```python
from build123d import *

# Parameters (mm, degrees)
SKETCH2_W           = 65
SKETCH2_H           = 65
BOSS_EXTRUDE1_DEPTH = 7
SKETCH3_R           = 5
BOSS_EXTRUDE2_DEPTH = 15
SKETCH4_R           = 4
CUT_EXTRUDE1_DEPTH  = 49.347699015


with BuildPart() as part:
    # Sketch2 → Boss-Extrude1 (new body)
    with BuildSketch(Plane.XY):
        Rectangle(SKETCH2_W, SKETCH2_H)
    extrude(amount=BOSS_EXTRUDE1_DEPTH)

    # Sketch3 → Boss-Extrude2 (add)
    with BuildSketch(Plane.XY.offset(7)):
        with Locations(Location((0, 0, 0), (0, 0, 180))):
            Circle(SKETCH3_R)
    extrude(amount=BOSS_EXTRUDE2_DEPTH)

    # Sketch4 → Cut-Extrude1 (cut, through all)
    with BuildSketch(Plane.XY.offset(7)):
        with Locations((-27.162431983, 27.037591963)):
            Circle(SKETCH4_R)
    extrude(amount=-CUT_EXTRUDE1_DEPTH, mode=Mode.SUBTRACT)


solid = part.part
```
Source: CAD feature listing. Evaluate the final solid. Frame: model axes, mm. A direction names the side the tool comes from. Round coordinates to 2 decimals unless told otherwise and drop trailing zeros. Order: outer loops, then holes, each group sorted by start corner. A loop starts at its lowest first (then second) coordinate and runs counter-clockwise, first axis right, second up. Notation, with made-up numbers: (72, 40) -> (107, 40) arc R16 cw to (107, 50) -> close; hole circle Ø7 at (69, 48). An arc over 180 degrees is marked (long way). One line per item, written item: value. Start each with the question number.
Q1. Section query C-C (x = -27). Return the cut outline in (y, z).
Q2. Material intervals for probe 1 along Z at (x, y) = (-19, -26); probe 2 along X at (y, z) = (24, 4.5); probe 3 along X at (y, z) = (4, 17.5), sorted ascending.
Q3. Pin query (flat end, axial travel): pin 1 (5 mm diameter, centred on x = 9, y = -2, fed in from +Z). Return the tip coordinate at first contact, or that it passes through.
Q4. Section query B-B (y = 24). Return the cut outline in (x, z), plus the area to 3 significant figures.
Q5. Section query A-A (x = 0). Return the cut outline in (y, z), plus the area to 3 significant figures.
Q6. Draft query along Y for faces 1 (the cylindrical face through (-27.7, 31, 3.5)), 2 (the flat face through (0, -32.5, 3)), 3 (the flat face through (0, -7, 7)). Return one class per face: pulls with the +Y half, pulls with the -Y half, needs draft (parallel to the pull), parting line crosses it, or undercut.
Q7. Access query for faces 4 (the cylindrical face through (5, 0, 14)), 5 (the flat face through (32.5, 0, 3)). Directions: +Z, -Z, +X, -X, +Y, -Y. A direction counts if a zero-diameter tool reaches every point of the face in a straight line with its end or side. Return the directions, or none.
Findings below:
1. outline: (-32.5, 0) -> (23.04, 0) -> (23.04, 7) -> (-32.5, 7) -> close; (31.03, 0) -> (32.5, 0) -> (32.5, 7) -> (31.03, 7) -> close
2. probe 1: 0 to 7
2. probe 2: -32.5 to -29.76, -24.56 to 32.5
2. probe 3: -3 to 3
3. pin 1: z = 7
4. outline: (-32.5, 0) -> (-29.76, 0) -> (-29.76, 7) -> (-32.5, 7) -> close; (-24.56, 0) -> (32.5, 0) -> (32.5, 7) -> (-24.56, 7) -> close
4. area: 419 mm²
5. outline: (-32.5, 0) -> (32.5, 0) -> (32.5, 7) -> (5, 7) -> (5, 22) -> (-5, 22) -> (-5, 7) -> (-32.5, 7) -> close
5. area: 605 mm²
6. face 1: undercut
6. face 2: pulls with the -Y half
6. face 3: needs draft
7. face 4: +Z
7. face 5: +Z, -Z, +X, +Y, -Y
